```python
from build123d import *

# Parameters (mm, degrees)
SKETCH1_R           = 2.5
BOSS_EXTRUDE1_DEPTH = 10
SKETCH2_R           = 2.5
BOSS_EXTRUDE2_DEPTH = 10
SKETCH3_R           = 5
SKETCH3_R_2         = 2.5
BOSS_EXTRUDE3_DEPTH = 6
SKETCH4_R           = 2.5
CUT_EXTRUDE1_DEPTH  = 6


with BuildPart() as part:
    # Sketch1 → Boss-Extrude1 (new body)
    with BuildSketch(Plane(origin=(4.043870029, 0, 0), x_dir=(0, 0, -1), z_dir=(1, 0, 0))):
        with BuildLine():
            ThreePointArc((-10.029541992, 0.342879069), (-9.019080639, -0.304016541), (-7.862233613, -0.622153359))
            ThreePointArc((-7.862233613, -0.622153359), (-7.876528296, -1.122077366), (-7.862233613, -1.622001374))
            ThreePointArc((-7.862233613, -1.622001374), (-9.019080639, -1.940138191), (-10.029541992, -2.587033801))
            ThreePointArc((-10.029541992, -2.587033801), (-9.992100042, -2.842856482), (-9.948655897, -3.097728508))
            ThreePointArc((-9.948655897, -3.097728508), (-8.787748306, -3.400713063), (-7.58921172, -3.345793765))
            ThreePointArc((-7.58921172, -3.345793765), (-7.448321757, -3.82566705), (-7.280241692, -4.296705735))
            ThreePointArc((-7.280241692, -4.296705735), (-8.282158911, -4.956757219), (-9.043263028, -5.884241235))
            ThreePointArc((-9.043263028, -5.884241235), (-8.928600062, -6.115972863), (-8.808522437, -6.344945585))
            ThreePointArc((-8.808522437, -6.344945585), (-7.610806331, -6.274360846), (-6.487901298, -5.851761317))
            ThreePointArc((-6.487901298, -5.851761317), (-6.20561798, -6.264610538), (-5.90020538, -6.660655353))
            ThreePointArc((-5.90020538, -6.660655353), (-6.649118154, -7.598011066), (-7.086362862, -8.715294889))
            ThreePointArc((-7.086362862, -8.715294889), (-6.905702889, -8.900251959), (-6.720745819, -9.080911932))
            ThreePointArc((-6.720745819, -9.080911932), (-5.603461996, -8.643667224), (-4.666106283, -7.89475445))
            ThreePointArc((-4.666106283, -7.89475445), (-4.270061468, -8.20016705), (-3.857212247, -8.482450368))
            ThreePointArc((-3.857212247, -8.482450368), (-4.279811776, -9.605355401), (-4.350396515, -10.803071507))
            ThreePointArc((-4.350396515, -10.803071507), (-4.121423793, -10.923149132), (-3.889692165, -11.037812099))
            ThreePointArc((-3.889692165, -11.037812099), (-2.962208149, -10.276707981), (-2.302156665, -9.274790762))
            ThreePointArc((-2.302156665, -9.274790762), (-1.83111798, -9.442870827), (-1.351244695, -9.583760791))
            ThreePointArc((-1.351244695, -9.583760791), (-1.406163992, -10.782297376), (-1.103179437, -11.943204968))
            ThreePointArc((-1.103179437, -11.943204968), (-0.848307411, -11.986649113), (-0.592484731, -12.024091063))
            ThreePointArc((-0.592484731, -12.024091063), (0.054410879, -11.01362971), (0.372547697, -9.856782684))
            ThreePointArc((0.372547697, -9.856782684), (0.872471704, -9.871077366), (1.372395712, -9.856782684))
            ThreePointArc((1.372395712, -9.856782684), (1.690532529, -11.01362971), (2.337428139, -12.024091063))
            ThreePointArc((2.337428139, -12.024091063), (2.59325082, -11.986649113), (2.848122846, -11.943204968))
            ThreePointArc((2.848122846, -11.943204968), (3.151107401, -10.782297376), (3.096188103, -9.583760791))
            ThreePointArc((3.096188103, -9.583760791), (3.576061388, -9.442870827), (4.047100073, -9.274790762))
            ThreePointArc((4.047100073, -9.274790762), (4.707151558, -10.276707981), (5.634635573, -11.037812099))
            ThreePointArc((5.634635573, -11.037812099), (5.866367201, -10.923149132), (6.095339923, -10.803071507))
            ThreePointArc((6.095339923, -10.803071507), (6.024755184, -9.605355401), (5.602155655, -8.482450368))
            ThreePointArc((5.602155655, -8.482450368), (6.015004877, -8.20016705), (6.411049691, -7.89475445))
            ThreePointArc((6.411049691, -7.89475445), (7.348405404, -8.643667224), (8.465689227, -9.080911932))
            ThreePointArc((8.465689227, -9.080911932), (8.650646297, -8.900251959), (8.83130627, -8.715294889))
            ThreePointArc((8.83130627, -8.715294889), (8.394061563, -7.598011066), (7.645148788, -6.660655353))
            ThreePointArc((7.645148788, -6.660655353), (7.950561388, -6.264610538), (8.232844706, -5.851761317))
            ThreePointArc((8.232844706, -5.851761317), (9.355749739, -6.274360846), (10.553465846, -6.344945585))
            ThreePointArc((10.553465846, -6.344945585), (10.67354347, -6.115972863), (10.788206437, -5.884241235))
            ThreePointArc((10.788206437, -5.884241235), (10.02710232, -4.956757219), (9.0251851, -4.296705735))
            ThreePointArc((9.0251851, -4.296705735), (9.193265165, -3.82566705), (9.334155129, -3.345793765))
            ThreePointArc((9.334155129, -3.345793765), (10.532691714, -3.400713063), (11.693599306, -3.097728508))
            ThreePointArc((11.693599306, -3.097728508), (11.737043451, -2.842856482), (11.774485401, -2.587033801))
            ThreePointArc((11.774485401, -2.587033801), (10.764024048, -1.940138191), (9.607177022, -1.622001374))
            ThreePointArc((9.607177022, -1.622001374), (9.621471704, -1.122077366), (9.607177022, -0.622153359))
            ThreePointArc((9.607177022, -0.622153359), (10.764024048, -0.304016541), (11.774485401, 0.342879069))
            ThreePointArc((11.774485401, 0.342879069), (11.737043451, 0.598701749), (11.693599306, 0.853573775))
            ThreePointArc((11.693599306, 0.853573775), (10.532691714, 1.156558331), (9.334155129, 1.101639033))
            ThreePointArc((9.334155129, 1.101639033), (9.193265165, 1.581512318), (9.0251851, 2.052551003))
            ThreePointArc((9.0251851, 2.052551003), (10.02710232, 2.712602487), (10.788206437, 3.640086503))
            ThreePointArc((10.788206437, 3.640086503), (10.67354347, 3.871818131), (10.553465846, 4.100790853))
            ThreePointArc((10.553465846, 4.100790853), (9.355749739, 4.030206114), (8.232844706, 3.607606585))
            ThreePointArc((8.232844706, 3.607606585), (7.950561388, 4.020455806), (7.645148788, 4.416500621))
            ThreePointArc((7.645148788, 4.416500621), (8.394061563, 5.353856334), (8.83130627, 6.471140157))
            ThreePointArc((8.83130627, 6.471140157), (8.650646297, 6.656097227), (8.465689227, 6.8367572))
            ThreePointArc((8.465689227, 6.8367572), (7.348405404, 6.399512492), (6.411049691, 5.650599718))
            ThreePointArc((6.411049691, 5.650599718), (6.015004877, 5.956012318), (5.602155655, 6.238295636))
            ThreePointArc((5.602155655, 6.238295636), (6.024755184, 7.361200669), (6.095339923, 8.558916775))
            ThreePointArc((6.095339923, 8.558916775), (5.866367201, 8.6789944), (5.634635573, 8.793657366))
            ThreePointArc((5.634635573, 8.793657366), (4.707151558, 8.032553249), (4.047100073, 7.03063603))
            ThreePointArc((4.047100073, 7.03063603), (3.576061388, 7.198716095), (3.096188103, 7.339606058))
            ThreePointArc((3.096188103, 7.339606058), (3.151107401, 8.538142644), (2.848122846, 9.699050235))
            ThreePointArc((2.848122846, 9.699050235), (2.59325082, 9.74249438), (2.337428139, 9.779936331))
            ThreePointArc((2.337428139, 9.779936331), (1.690532529, 8.769474978), (1.372395712, 7.612627952))
            ThreePointArc((1.372395712, 7.612627952), (0.872471704, 7.626922634), (0.372547697, 7.612627952))
            ThreePointArc((0.372547697, 7.612627952), (0.054410879, 8.769474978), (-0.592484731, 9.779936331))
            ThreePointArc((-0.592484731, 9.779936331), (-0.848307411, 9.74249438), (-1.103179437, 9.699050235))
            ThreePointArc((-1.103179437, 9.699050235), (-1.406163992, 8.538142644), (-1.351244695, 7.339606058))
            ThreePointArc((-1.351244695, 7.339606058), (-1.83111798, 7.198716095), (-2.302156665, 7.03063603))
            ThreePointArc((-2.302156665, 7.03063603), (-2.962208149, 8.032553249), (-3.889692165, 8.793657366))
            ThreePointArc((-3.889692165, 8.793657366), (-4.121423793, 8.6789944), (-4.350396515, 8.558916775))
            ThreePointArc((-4.350396515, 8.558916775), (-4.279811776, 7.361200669), (-3.857212247, 6.238295636))
            ThreePointArc((-3.857212247, 6.238295636), (-4.270061468, 5.956012318), (-4.666106283, 5.650599718))
            ThreePointArc((-4.666106283, 5.650599718), (-5.603461996, 6.399512492), (-6.720745819, 6.8367572))
            ThreePointArc((-6.720745819, 6.8367572), (-6.905702889, 6.656097227), (-7.086362862, 6.471140157))
            ThreePointArc((-7.086362862, 6.471140157), (-6.649118154, 5.353856334), (-5.90020538, 4.416500621))
            ThreePointArc((-5.90020538, 4.416500621), (-6.20561798, 4.020455806), (-6.487901298, 3.607606585))
            ThreePointArc((-6.487901298, 3.607606585), (-7.610806331, 4.030206114), (-8.808522437, 4.100790853))
            ThreePointArc((-8.808522437, 4.100790853), (-8.928600062, 3.871818131), (-9.043263028, 3.640086503))
            ThreePointArc((-9.043263028, 3.640086503), (-8.282158911, 2.712602487), (-7.280241692, 2.052551003))
            ThreePointArc((-7.280241692, 2.052551003), (-7.448321757, 1.581512318), (-7.58921172, 1.101639033))
            ThreePointArc((-7.58921172, 1.101639033), (-8.787748306, 1.156558331), (-9.948655897, 0.853573775))
            ThreePointArc((-9.948655897, 0.853573775), (-9.992100042, 0.598701749), (-10.029541992, 0.342879069))
        make_face()
        with Locations(Location((0.872471704, -1.122077366, 0), (0, 0, 180))):
            Circle(SKETCH1_R, mode=Mode.SUBTRACT)
    extrude(amount=-BOSS_EXTRUDE1_DEPTH)

    # Sketch2 → Boss-Extrude2 (add)
    with BuildSketch(Plane(origin=(4.043870029, 0, 0), x_dir=(0, 0, -1), z_dir=(1, 0, 0))):
        with BuildLine():
            Line((0.872471704, 3.877922634), (30.872471704, 3.877922634))
            ThreePointArc((30.872471704, 3.877922634), (35.872471704, -1.122077366), (30.872471704, -6.122077366))
            Line((30.872471704, -6.122077366), (0.872471704, -6.122077366))
            ThreePointArc((0.872471704, -6.122077366), (-4.127528296, -1.122077366), (0.872471704, 3.877922634))
        make_face()
        with Locations((30.872471704, -1.122077366)):
            Circle(SKETCH2_R, mode=Mode.SUBTRACT)
    extrude(amount=-BOSS_EXTRUDE2_DEPTH)

    # Sketch3 → Boss-Extrude3 (add)
    with BuildSketch(Plane.ZY.offset(5.956129971)):
        with Locations(Location((-30.872471704, -1.122077366, 0), (0, 0, 270))):
            Circle(SKETCH3_R)
        with Locations(Location((-30.872471704, -1.122077366, 0), (0, 0, 180))):
            Circle(SKETCH3_R_2, mode=Mode.SUBTRACT)
    extrude(amount=BOSS_EXTRUDE3_DEPTH)

    # Sketch4 → Cut-Extrude1 (cut)
    with BuildSketch(Plane(origin=(4.043870029, 0, 0), x_dir=(0, 0, -1), z_dir=(1, 0, 0))):
        with Locations((0.872471704, -1.122077366)):
            Circle(SKETCH4_R)
    extrude(amount=-CUT_EXTRUDE1_DEPTH, mode=Mode.SUBTRACT)


solid = part.part
```
Could you check a few things on this model? Use its own coordinates, in mm. A direction names the side the tool comes from. Round coordinates to 2 decimals unless told otherwise and drop trailing zeros. Write each loop counter-clockwise with the first axis right and the second up, starting at its lowest first coordinate (ties: lowest second). Pieces come first, ordered by that corner, then holes.
(1) Which directions (+Z, -Z, +X, -X, +Y, -Y) give clear straight access to the entire face, cutting with the end or side of a thin tool? Please do faces 4 (the face through (-0.89, 6.39, 5.59)), 5 (the face through (-0.886, -10.264, -4.696)), 6 (the face through (-0.886, -9.589, 4.276)), 7 (the face through (-1, -6.122, -21)).
Findings below:
face 4: +X, -X, +Y
face 5: +X, -X, -Y
face 6: +X, -X
face 7: -Z, +X, -X, -Y
(2) Suppose I cut it at A-A on z = -30. Write out the boundary of the cut face in (x, y).
Findings below:
outline: (-11.96, -6.05) - (-5.96, -6.05) - (-5.96, -6.12) - (4.04, -6.12) - (4.04, -3.46) - (-11.96, -3.46) - close; (-11.96, 1.22) - (4.04, 1.22) - (4.04, 3.88) - (-5.96, 3.88) - (-5.96, 3.8) - (-11.96, 3.8) - close
(3) If I drill on probe 1 along Z at (x, y) = (3, -1.25); probe 2 along Y at (x, z) = (-4, -8); probe 3 along Z at (x, y) = (1, 0), over which ranges is the centre line in solid material (lowest first)?
Findings below:
probe 1: z = -35.87 to -33.37, -28.38 to -3.37, 1.62 to 7.88
probe 2: y = -8.95 to -7.03, -6.2 to 3.95, 4.79 to 6.7
probe 3: z = -35.74 to -33.11, -28.64 to -3.11, 1.36 to 9.58
(4) Suppose I cut it at D-D on x = -0.5. State how many separate pieces and enclosed holes the cut face has, and give its area (3 significant figures).
Findings below:
separate pieces: 1
enclosed holes: 2
area: 508 mm2
(5) For pin 1 (1 mm diameter, centred on x = -4, y = 6.5, fed in from -Z); pin 2 (0.8 mm diameter, centred on x = 0, z = -8.5, fed in from +Y); pin 3 (12 mm diameter, centred on y = -6.5, z = -18, fed in from -X), each with a flat end and sliding along its axis, tell me the tip position at first contact or that it passes through.
Findings below:
pin 1: stops at z = -8.83
pin 2: stops at y = 6.84
pin 3: stops at x = -5.96
(6) Suppose I cut it at B-B on x = -10.25. Write out the boundary of the cut face in (y, z).
Findings below:
outline: circle Ø10 at (-1.12, -30.87); hole circle Ø5 at (-1.12, -30.87)
(7) Suppose I cut it at C-C on z = -18. Write out the boundary of the cut face in (x, y), and give its area (3 significant figures).
Findings below:
outline: (-5.96, -6.12) - (4.04, -6.12) - (4.04, 3.88) - (-5.96, 3.88) - close
area: 100 mm2
(8) Thinking about a two-plate mould opening in Y: for faces 1 (the face through (-0.89, 5.95, -6.02)), 2 (the face through (-0.886, -10.998, -1.684)), 3 (the face through (-1, 3.878, -21)), which applies, +Y half, -Y half, draft (parallel to the pull), parting line (faces both ways), or undercut?
Findings below:
face 1: undercut
face 2: -Y half
face 3: +Y half
